CAD build for the part. Positions are in the model's coordinates, mm. Face numbers are marked on the shaded views. Give positions to 0.01 mm unless a question says otherwise; leave off trailing zeros. Loops run counter-clockwise (first coordinate to the right, second up) from the corner with the lowest first, then second, coordinate; pieces in that order, holes last. Notation, with made-up numbers: (86, 86) -> (133, 86) arc R28 ccw to (133, 117) -> close; hole circle Ø3 at (9, 32). An arc over 180 degrees is marked (long way). Use one line per item in the form item = value.
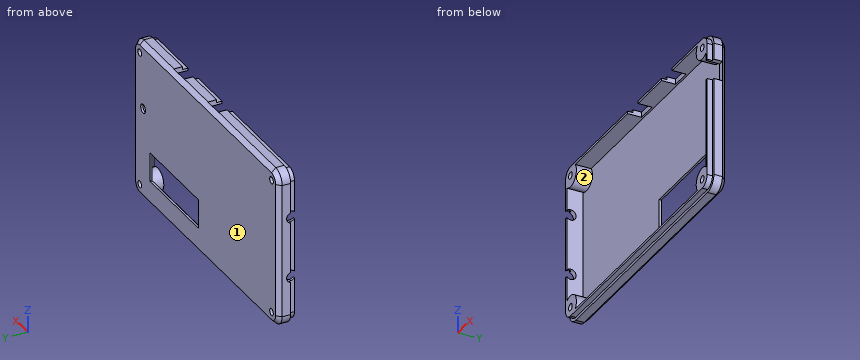
```python
from build123d import *

# Parameters (mm, degrees)
CYLINDER001_R           = 2
CYLINDER001_DEPTH       = 10
SKETCH037_W             = 7.5
SKETCH037_H             = 7.5
EXTRUDE045_DEPTH        = 10
BOX089_W                = 11
BOX089_H                = 10
BOX089_DEPTH            = 35
BODY005_PLACEMENT_ANGLE = 90
BODY006_PLACEMENT_ANGLE = 90
CYLINDER003_R           = 2
CYLINDER003_DEPTH       = 10
CYLINDER002_R           = 1.7
CYLINDER002_DEPTH       = 10
SKETCH005_R             = 1.3
EXTRUDE003_DEPTH        = 20
EXTRUDE039_DEPTH        = 4
EXTRUDE042_DEPTH        = 0.8
EXTRUDE002_DEPTH        = 6
EXTRUDE037_DEPTH        = 2


with BuildPart() as battery_cable:
    # Cylinder001 → Cylinder001 (new body)
    with BuildSketch(Plane(origin=(-66.5, 0, 35), x_dir=(0, 0, 1), z_dir=(-1, 0, 0))):
        Circle(CYLINDER001_R)
    extrude(amount=CYLINDER001_DEPTH)


with BuildPart() as switch_hole002:
    # Sketch037 → Extrude045 (new body)
    with BuildSketch(Plane.YZ.offset(35)):
        with Locations((0, 38.5)):
            Rectangle(SKETCH037_W, SKETCH037_H)
    extrude(amount=EXTRUDE045_DEPTH)


with BuildPart() as switch_hole002_1:
    # Extrude045 placement: moved
    add(switch_hole002.part.moved(Location((-9.5, 0, 0))))


with BuildPart() as dips001:
    # Box089 → Box089 (new body)
    with BuildSketch(Plane(origin=(-15, 0.5, 13.5), x_dir=(0, 0, -1), z_dir=(1, 0, 0))):
        with Locations((5.5, 5)):
            Rectangle(BOX089_W, BOX089_H)
    extrude(amount=BOX089_DEPTH)


with BuildPart() as switch_hole001:
    # Body005 base: copy of switch hole002
    add(switch_hole002_1.part)


with BuildPart() as switch_hole001_1:
    # Body005 placement: moved
    add(switch_hole001.part.moved(Location((40.5, 0, 22))).rotate(Axis((40.5, 0, 22), (0, -1, 0)), BODY005_PLACEMENT_ANGLE))


with BuildPart() as switch_hole:
    # Body006 base: copy of switch hole002
    add(switch_hole002_1.part)


with BuildPart() as switch_hole_1:
    # Body006 placement: moved
    add(switch_hole.part.moved(Location((16, 0, 22))).rotate(Axis((16, 0, 22), (0, -1, 0)), BODY006_PLACEMENT_ANGLE))


with BuildPart() as cable:
    # Cylinder003 → Cylinder003 (new body)
    with BuildSketch(Plane(origin=(-65.5, 0, 12), x_dir=(0, -1, 0), z_dir=(-1, 0, 0))):
        Circle(CYLINDER003_R)
    extrude(amount=CYLINDER003_DEPTH)


with BuildPart() as common_sub:
    # Cylinder002 → Cylinder002 (new body)
    with BuildSketch(Plane(origin=(25, -1.5, 28), x_dir=(1, 0, 0), z_dir=(0, 1, 0))):
        Circle(CYLINDER002_R)
    extrude(amount=CYLINDER002_DEPTH)

    # Fusion033: union battery cable, switch hole002, dips001, switch hole001, switch hole, cable
    add(battery_cable.part)
    add(switch_hole002_1.part)
    add(dips001.part)
    add(switch_hole001_1.part)
    add(switch_hole_1.part)
    add(cable.part)


with BuildPart() as sweep001:
    # Sweep001: sweep along a path in Sketch034
    with BuildLine(Plane.XZ.offset(10)) as sweep001_path:
        Line((32, 12), (32, 48.4))
        ThreePointArc((32, 48.4), (30.652691, 51.652691), (27.4, 53))
        Line((27.4, 53), (-20, 53))
    # Sketch035 → Sweep001 (sweep)
    with BuildSketch(Plane.YZ):
        Polygon((5.3, 51.4), (3.7, 53), (3.7, 54), (6, 54), (6, 51.4), align=None)
    sweep(path=sweep001_path.line)


with BuildPart() as fusion030:
    # Sketch005 → Extrude003 (new body)
    with BuildSketch(Plane.XZ.offset(5)):
        with Locations((27.4, 48.5)):
            Circle(SKETCH005_R)
    extrude(amount=-EXTRUDE003_DEPTH)


with BuildPart() as fusion030_1:
    # Extrude003 placement: moved
    add(fusion030.part.moved(Location((0, -4, 0))))

    # Fusion030: union Sweep001
    add(sweep001.part)


with BuildPart() as top003:
    # Sketch028 → Extrude039 (new body)
    with BuildSketch(Plane.XZ.offset(10)):
        with BuildLine():
            ThreePointArc((32, 48.4), (30.652691, 51.652691), (27.4, 53))
            Line((27.4, 53), (-20, 53))
            Line((-20, 53), (-20, 51))
            Line((-20, 51), (27.4, 51))
            ThreePointArc((30, 48.4), (29.238478, 50.238478), (27.4, 51))
            Line((30, 23), (30, 48.4))
            Line((32, 23), (30, 23))
            Line((32, 48.4), (32, 23))
        make_face()
    extrude(amount=EXTRUDE039_DEPTH)


with BuildPart() as top003_1:
    # Extrude039 placement: moved
    add(top003.part.moved(Location((0, 14.5, 0))))


with BuildPart() as top002:
    # Sketch031 → Extrude042 (new body)
    with BuildSketch(Plane.XZ.offset(10)):
        with BuildLine():
            ThreePointArc((32, 48.4), (30.652691, 51.652691), (27.4, 53))
            Line((27.4, 53), (-20, 53))
            Line((-20, 53), (-20, 23))
            Line((-20, 23), (32, 23))
            Line((32, 48.4), (32, 23))
        make_face()
    extrude(amount=EXTRUDE042_DEPTH)


with BuildPart() as top002_1:
    # Extrude042 placement: moved
    add(top002.part.moved(Location((0, 15.3, 0))))


with BuildPart() as screw_hole_top:
    # Sketch004 → Extrude002 (new body)
    with BuildSketch(Plane.XZ.offset(10)):
        with BuildLine():
            ThreePointArc((23.975091, 51), (24.359441, 45.359441), (30, 44.975091))
            Line((30, 44.975091), (30, 48.4))
            ThreePointArc((30, 48.4), (29.238478, 50.238478), (27.4, 51))
            Line((23.975091, 51), (27.4, 51))
        make_face()
    extrude(amount=-EXTRUDE002_DEPTH)


with BuildPart() as screw_hole_top_1:
    # Extrude002 placement: moved
    add(screw_hole_top.part.moved(Location((0, 8.5, 0))))


with BuildPart() as top:
    # Sketch029 → Extrude037 (new body)
    with BuildSketch(Plane.XZ.offset(10)):
        with BuildLine():
            ThreePointArc((30.9, 48.4), (29.874874, 50.874874), (27.4, 51.9))
            Line((27.4, 51.9), (-20, 51.9))
            Line((-20, 51.9), (-20, 51))
            Line((-20, 51), (27.4, 51))
            ThreePointArc((30, 48.4), (29.238478, 50.238478), (27.4, 51))
            Line((30, 23), (30, 48.4))
            Line((30.9, 23), (30, 23))
            Line((30.9, 48.4), (30.9, 23))
        make_face()
    extrude(amount=EXTRUDE037_DEPTH)


with BuildPart() as top_1:
    # Extrude037 placement: moved
    add(top.part.moved(Location((0, 10.5, 0))))

    # Fusion028: union top003, top002, screw hole top
    add(top003_1.part)
    add(top002_1.part)
    add(screw_hole_top_1.part)

    # Cut024: cut Fusion030
    add(fusion030_1.part, mode=Mode.SUBTRACT)


with BuildPart() as part_mirroring:
    # Part__Mirroring: instance of top
    add(top_1.part.mirror(Plane(origin=(0, 0, 23), x_dir=(0, 1, 0), z_dir=(0, 0, 1))))


with BuildPart() as part_mirroring002:
    # Part__Mirroring002: instance of Part__Mirroring
    add(part_mirroring.part.mirror(Plane(origin=(-20, 1, 0), x_dir=(0, -1, 0), z_dir=(1, 0, 0))))


with BuildPart() as top007:
    # Part__Mirroring003: instance of top
    add(top_1.part.mirror(Plane(origin=(-20, 0, 0), x_dir=(0, -1, 0), z_dir=(1, 0, 0))))

    # Fusion032: union top, Part__Mirroring, Part__Mirroring002
    add(top_1.part)
    add(part_mirroring.part)
    add(part_mirroring002.part)

    # Cut025: cut common sub
    add(common_sub.part, mode=Mode.SUBTRACT)


solid = top007.part
```
1. Cut at A-A, the plane z = 5. Write the cut outline in (x, y), then the cut area to 3 significant figures.
Result sheet:
outline = (-72, 0.5) -> (-70.9, 0.5) -> (-70.9, -1.5) -> (-70, -1.5) -> (-70, 4.5) -> (-15, 4.5) -> (-15, 5.3) -> (-70.4, 5.3) -> (-72, 3.7) -> close; (20, 4.5) -> (30, 4.5) -> (30, -1.5) -> (30.9, -1.5) -> (30.9, 0.5) -> (32, 0.5) -> (32, 3.7) -> (30.4, 5.3) -> (20, 5.3) -> close
area = 72.2 mm^2
2. Drill centre lines: line 1 (X direction, y = 1.75, z = -2.5); line 2 (Z direction, x = -67.4, y = 1.5); line 3 (Z direction, x = -47.5, y = -1). Where is each one in solid material? Low to high.
Result sheet:
line_1 = -72 to -68.7, -66.1 to -63.1, 23.1 to 26.1, 28.7 to 32
line_2 = -7 to -3.8, -1.2 to 1.9, 44.1 to 47.2, 49.8 to 53
line_3 = -5.9 to -5, 51 to 51.9
3. Drop flat-ended pins along their axis: P1, Ø2, axis at x = -22.5, z = 52, coming from the -Y side; P2, Ø12.5, axis at x = -26, z = 10.5, coming from the -Y side; P3, Ø0.6, axis at y = 1, z = 51.5, coming from the -X side. Give the stop position or say it passes through.
Result sheet:
P1 = 3.75
P2 = 4.5
P3 = -71.05
4. Cut at C-C, the plane x = -25. Write the cut outline in (y, z), then the cut area to 3 significant figures.
Result sheet:
outline = (-1.5, -5.9) -> (0.5, -5.9) -> (0.5, -7) -> (3.7, -7) -> (5.3, -5.4) -> (5.3, 51.4) -> (3.75, 52.95) -> (3.75, 51) -> (4.5, 51) -> (4.5, -5) -> (-1.5, -5) -> close
area = 56.7 mm^2
5. Mould opens along X. For the marked faces 1 and 2 say: pulls with the +X half, pulls with the -X half, needs draft (parallel to the pull), parting line crosses it, or undercut.
Result sheet:
face_1 = needs draft
face_2 = undercut
6. Cut at D-D, the plane z = 17. Write the cut outline in (x, y), then the cut area to 3 significant figures.
Result sheet:
outline = (-72, 0.5) -> (-70.9, 0.5) -> (-70.9, -1.5) -> (-70, -1.5) -> (-70, 4.5) -> (30, 4.5) -> (30, -1.5) -> (30.9, -1.5) -> (30.9, 0.5) -> (32, 0.5) -> (32, 3.7) -> (30.4, 5.3) -> (-70.4, 5.3) -> (-72, 3.7) -> close
area = 100 mm^2
7. Cut at B-B, the plane x = 3. Write the cut outline in (y, z), then the cut area to 3 significant figures.
Result sheet:
outline = (-1.5, -5.9) -> (0.5, -5.9) -> (0.5, -7) -> (3.7, -7) -> (5.3, -5.4) -> (5.3, 2.5) -> (4.5, 2.5) -> (4.5, -5) -> (-1.5, -5) -> close; (3.75, 51) -> (4.5, 51) -> (4.5, 13.5) -> (5.3, 13.5) -> (5.3, 51.4) -> (3.75, 52.95) -> close
area = 47.9 mm^2
